Autodesk Inventor part; units mm, degrees
ref_plane "YZ Plane" through (0, 0, 0) normal (1, 0, 0) x (0, 1, 0)
ref_plane "XZ Plane" through (0, 0, 0) normal (0, 1, 0) x (-1, 0, 0)
ref_plane "XY Plane" through (0, 0, 0) normal (0, 0, 1) x (1, 0, 0)
sketch "Sketch1" plane through (0, 0, 0) normal (0, 0, 1) x (1, 0, 0)
  line L0 (0, 225) -> (0, -225)
  line L1 (0, -225) -> (-700, -225)
  line L2 (-700, -225) -> (-700, 225)
  line L3 (-700, 225) -> (0, 225)
  point P0 (0, 0)
extrude "Extrusion1" add sketch "Sketch1" along normal blind 30
sketch "Sketch2" plane through (0, 0, 30) normal (0, 0, 1) x (1, 0, 0)
  line L0 (0, -225) -> (-700, -225)
  line L1 (0, 225) -> (0, -225)
  line L2 (-700, 225) -> (0, 225)
  line L3 (-700, -225) -> (-700, 225)
  line L4 (-15, 210) -> (-15, -210)
  line L5 (-15, -210) -> (-685, -210)
  line L6 (-685, -210) -> (-685, 210)
  line L7 (-685, 210) -> (-15, 210)
  point P0 (0, 0)
  dimension "d2" = 15
extrude "Extrusion2" cut sketch "Sketch2" against normal blind 3 contours L4 L5 L6 L7
sketch "Sketch3" plane through (0, 0, 27) normal (0, 0, 1) x (1, 0, 0)
  line L0 (-15, 210) -> (-685, 210)
  line L1 (-685, 210) -> (-685, -210)
  line L2 (-685, -210) -> (-15, -210)
  line L3 (-525, 210) -> (-525, -210)
  point P0 (0, 0)
  dimension "d5" = 160
extrude "Extrusion3" cut sketch "Sketch3" against normal blind 23.6375
properties part number "CatcherBox"
The model under review builds one solid part; all positions refer to its coordinate system, in mm. A direction names the side the tool comes from. Round coordinates to 2 decimals unless told otherwise and drop trailing zeros. Loops run counter-clockwise (first coordinate to the right, second up) from the corner with the lowest first, then second, coordinate; pieces in that order, holes last. Notation, with made-up numbers: M 77,-10 L 117,-10 A24 ccw 117,12 Z; hole C 12.5,24.25 d4. An arc over 180 degrees is marked long. Write item = value, one per line.
Item 1: The part is to be moulded in two halves that separate along Y. For faces 3 (the flat face through (-274, 3, 27)), 4 (the flat face through (0, 3, 15)), 5 (the flat face through (-355, 225, 15)), say which applies: released by +Y, released by -Y, zero draft, split by the parting line, or undercut.
Return value:
face_3 = undercut
face_4 = zero draft
face_5 = released by +Y
Item 2: Take a section at D-D on x = -592. Write out the cut boundary in (y, z), then the cut area to 3 significant figures.
Return value:
outline = M -225,0 L 225,0 L 225,30 L 210,30 L 210,3.36 L -210,3.36 L -210,30 L -225,30 Z
area = 2,310 mm2
Item 3: Take a section at C-C on x = -434. Write out the cut boundary in (y, z), then the cut area to 3 significant figures.
Return value:
outline = M -225,0 L 225,0 L 225,30 L 210,30 L 210,27 L -210,27 L -210,30 L -225,30 Z
area = 12,200 mm2
Item 4: Take a section at A-A on z = 18.5. Write out the cut boundary in (x, y).
Return value:
outline = M -700,-225 L 0,-225 L 0,225 L -700,225 Z; hole M -685,-210 L -525,-210 L -525,210 L -685,210 Z
Item 5: Insertion check: P1, Ø8, axis at x = -244.5, y = -59.5, coming from the +Z side. The pin has a flat end and moves straight along its axis. Give the tip position at first contact, or say it passes through.
Return value:
P1 = 27
Item 6: Machinability: for faces 1 (the flat face through (-522, -210, 28)), 2 (the flat face through (-700, -3, 15)), which of the approach directions +Z, -Z, +X, -X, +Y, -Y give a long, thin tool a straight path to every point of the face, cutting with its end or side? Answer none if there is none.
Return value:
face_1 = +Z
face_2 = +Z, -Z, -X, +Y, -Y
Item 7: For line 1 (X direction, y = -182.5, z = 8.25); line 2 (Y direction, x = -454, z = 28); line 3 (Z direction, x = -423.5, y = 23), list the stretches that pass through material, from the lowest coordinate up. Write a range as [from, to].
Return value:
line_1 = [-700, -685], [-525, 0]
line_2 = [-225, -210], [210, 225]
line_3 = [0, 27]
Item 8: Take a section at B-B on y = -188.5. Write out the cut boundary in (x, z), then the cut area to 3 significant figures.
Return value:
outline = M -700,0 L 0,0 L 0,30 L -15,30 L -15,27 L -525,27 L -525,3.36 L -685,3.36 L -685,30 L -700,30 Z
area = 15,200 mm2
